```python
from build123d import *

# Parameters (mm, degrees)
F0_R     = 3
F0_R_2   = 2
F1_DEPTH = 2


with BuildPart() as f1:
    # F0 (on Front) → F1 (new body)
    with BuildSketch(Plane.XZ):
        Polygon((-24.489924, 30), (-24.489924, 0), (45.510076, 0), (45.510076, 70), (35.510076, 70), align=None)
        with Locations((-8.489924, 17)):
            Circle(F0_R, mode=Mode.SUBTRACT)
        with Locations((26.510076, 17)):
            Circle(F0_R, mode=Mode.SUBTRACT)
        with Locations((39.510076, 64)):
            Circle(F0_R_2, mode=Mode.SUBTRACT)
    extrude(amount=F1_DEPTH)


solid = f1.part
```
The model under review builds one solid part; all positions refer to its coordinate system, in mm. Round coordinates to 2 decimals unless told otherwise and drop trailing zeros. Loops run counter-clockwise (first coordinate to the right, second up) from the corner with the lowest first, then second, coordinate; pieces in that order, holes last.
Item 1: For line 1 (Z direction, x = 24, y = -1.5); line 2 (Z direction, x = 25, y = -1.8); line 3 (X direction, y = -0.05, z = 15.5), list the stretches that pass through material, from the lowest coordinate up.
Determined:
line 1: z = 0 to 15.36, 18.64 to 62.33
line 2: z = 0 to 14.41, 19.59 to 62.99
line 3: x = -24.49 to -11.09, -5.89 to 23.91, 29.11 to 45.51
Item 2: Take a section at D-D (z = 64). Write out the cut boundary in (x, y).
Determined:
outline: (26.51, -2) - (37.51, -2) - (37.51, 0) - (26.51, 0) - close; (41.51, -2) - (45.51, -2) - (45.51, 0) - (41.51, 0) - close
Item 3: Take a section at C-C (x = -10.5). Write out the cut boundary in (y, z).
Determined:
outline: (-2, 0) - (0, 0) - (0, 14.77) - (-2, 14.77) - close; (-2, 19.23) - (0, 19.23) - (0, 39.33) - (-2, 39.33) - close
Item 4: Take a section at B-B (y = -1.35). Write out the cut boundary in (x, z).
Determined:
outline: (-24.49, 0) - (45.51, 0) - (45.51, 70) - (35.51, 70) - (-24.49, 30) - close; hole circle Ø6 at (-8.49, 17); hole circle Ø6 at (26.51, 17); hole circle Ø4 at (39.51, 64)
Item 5: Take a section at A-A (z = 17). Write out the cut boundary in (x, y), then the cut area to 3 significant figures.
Determined:
outline: (-24.49, -2) - (-11.49, -2) - (-11.49, 0) - (-24.49, 0) - close; (-5.49, -2) - (23.51, -2) - (23.51, 0) - (-5.49, 0) - close; (29.51, -2) - (45.51, -2) - (45.51, 0) - (29.51, 0) - close
area: 116 mm2
Item 6: Mouldability with a two-part tool opening along Z and no side actions: class faces 1 (the face through (40.585, -0.986, 65.686)), 2 (the face through (10, -1, 0)), 3 (the face through (18, -2, 28)) as released by +Z, released by -Z, zero draft, split by the parting line, or undercut.
Determined:
face 1: undercut
face 2: released by -Z
face 3: zero draft
